Print and shaded views of the part. All mm, measured from the part's lowest x, y and z. A direction names the side the tool comes from. Coordinates: 2 decimals unless noted, no trailing zeros. Loops run counter-clockwise (first coordinate to the right, second up) from the corner with the lowest first, then second, coordinate; pieces in that order, holes last. Notation, with made-up numbers: M 72,9.25 L 118,9.25 A28 ccw 118,27.25 Z; hole C 58.5,73 d10. An arc over 180 degrees is marked long. Use a Markdown table: item, result. Add a question column.
1) Band-saw the part on B-B (x = 4). List the corners of the cut face in (y, z), plus the area to 3 significant figures.
2) Tool access for the marked faces 1, 2, 3 and 4: list every direction of +Z, -Z, +X, -X, +Y, -Y with a clear straight run to the whole face (end or side of a thin tool).
3) Band-saw the part on A-A (z = 4). List the corners of the cut face in (x, y) (3 decimals).
4) Band-saw the part on C-C (y = 4). List the corners of the cut face in (x, z) (3 decimals), plus the area to 3 significant figures.
5) Wall check: probe 1 along X at (y, z) = (1, 11.75); probe 2 along Z at (x, y) = (5.5, 7.5); probe 3 along Y at (x, z) = (3.75, 3.75). Give the ranges that are in metal, low to high. Write a range as from..to.
6) Pull direction Y, two halves, no side cores. Call the marked faces 5, 6 and 7: released by +Y, released by -Y, zero draft, split by the parting line, or undercut.
7) Pin check, flat tips, straight feed: pin 1 Ø1 at (x, z) = (3.5, 5) entering from -Y; pin 2 Ø2 at (y, z) = (2, 5) entering from -X (3 decimals); pin 3 Ø1 at (x, z) = (6.5, 18) entering from -Y. Stop position of each tip, or through.
8) Band-saw the part on D-D (z = 9.75). List the corners of the cut face in (x, y).
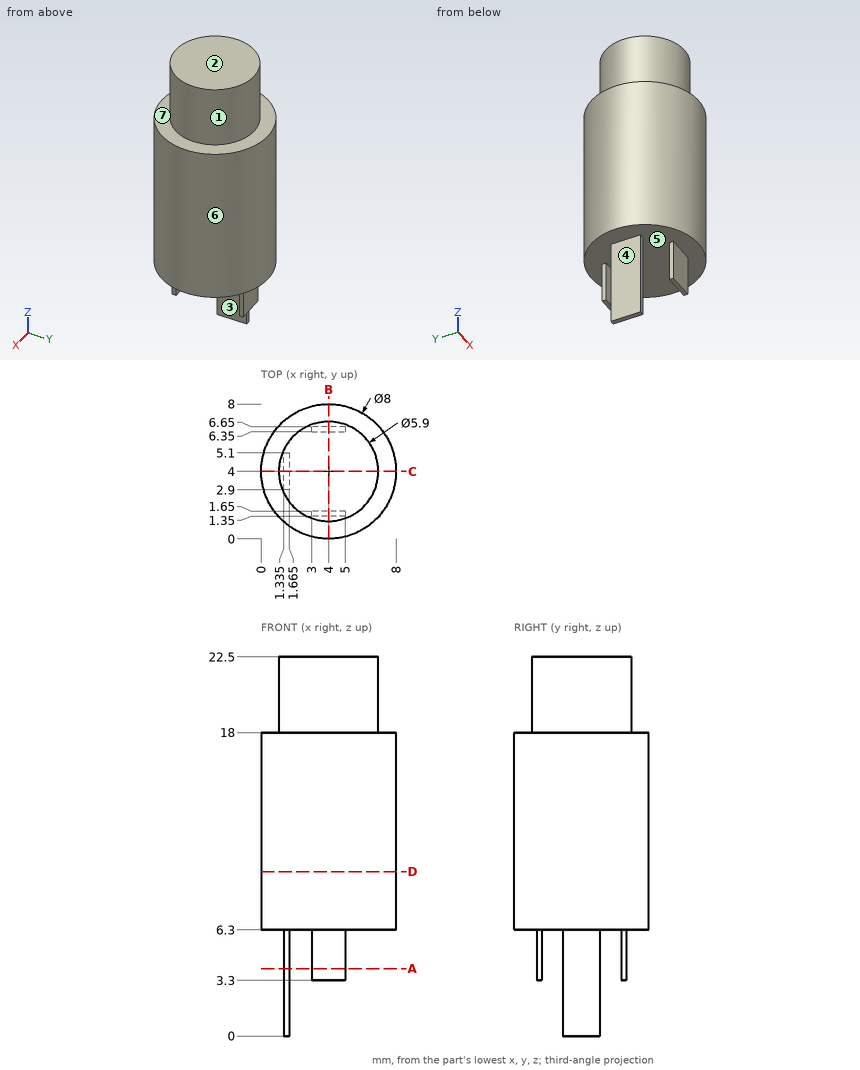
Entries:
| question | item | result |
|---|---|---|
| 1 | outline | M 0,6.3 L 1.35,6.3 L 1.35,3.3 L 1.65,3.3 L 1.65,6.3 L 6.35,6.3 L 6.35,3.3 L 6.65,3.3 L 6.65,6.3 L 8,6.3 L 8,18 L 6.95,18 L 6.95,22.5 L 1.05,22.5 L 1.05,18 L 0,18 Z |
| 1 | area | 122 mm2 |
| 2 | face 1 | +Z |
| 2 | face 2 | +Z, +X, -X, +Y, -Y |
| 2 | face 3 | -Z, +X, +Y, -Y |
| 2 | face 4 | -Z, -X, +Y, -Y |
| 3 | outline | M 1.335,2.9 L 1.665,2.9 L 1.665,5.1 L 1.335,5.1 Z; M 3,1.35 L 5,1.35 L 5,1.65 L 3,1.65 Z; M 3,6.35 L 5,6.35 L 5,6.65 L 3,6.65 Z |
| 4 | outline | M 0,6.3 L 1.335,6.3 L 1.335,0 L 1.665,0 L 1.665,6.3 L 8,6.3 L 8,18 L 6.95,18 L 6.95,22.5 L 1.05,22.5 L 1.05,18 L 0,18 Z |
| 4 | area | 122 mm2 |
| 5 | probe 1 | 1.35..6.65 |
| 5 | probe 2 | 6.3..18 |
| 5 | probe 3 | 1.35..1.65, 6.35..6.65 |
| 6 | face 5 | undercut |
| 6 | face 6 | split by the parting line |
| 6 | face 7 | zero draft |
| 7 | pin 1 | y = 1.35 |
| 7 | pin 2 | x = 1.335 |
| 7 | pin 3 | y = 0.54 |
| 8 | outline | C 4,4 d8 |
